Could you check a few things on this drawing? It's one solid part, dimensions in mm from its lowest x, y, z. A direction names the side the tool comes from. Coordinates: 2 decimals unless noted, no trailing zeros. Order: outer loops, then holes, each group sorted by start corner. A loop starts at its lowest first (then second) coordinate and runs counter-clockwise, first axis right, second up. Notation, with made-up numbers: (-6, 48.25) -> (1, 48.25) arc R21 ccw to (1, 58.25) -> close; hole circle Ø4 at (5.5, 3.25). An arc over 180 degrees is marked (long way). Use a Markdown table: item, result. Add a question column.
1. If I drill on line 1 along Z through (x, y) = (36.09, 1.05); line 2 along Y through (x, z) = (40, 22.5), over which ranges is the centre line in solid material (lowest first)? Write a range as from..to.
2. Suppose I cut it at D-D, the plane z = 22.5. List the corners of the cut face in (x, y) for me, then the cut area to 3 significant figures.
3. Suppose I cut it at A-A, the plane z = 6.28. List the corners of the cut face in (x, y) for me, then the cut area to 3 significant figures.
4. Suppose I cut it at C-C, the plane z = 26.5. List the corners of the cut face in (x, y) for me, then the cut area to 3 significant figures.
5. Suppose I cut it at B-B, the plane x = 36.09. List the corners of the cut face in (y, z) for me, then the cut area to 3 significant figures.
6. For pin 1 Ø5 at (x, z) = (19, 13.5) entering from -Y; pin 2 Ø1 at (y, z) = (23, 21) entering from +X; pin 3 Ø1.5 at (x, z) = (27.5, 5) entering from +Y, each with a flat end and sliding along its axis, tell me the tip position at first contact or that it passes through.
7. For the marked faces 1 and 2, which set-ups out of +Z, -Z, +X, -X, +Y, -Y let a thin tool reach every point of the face, with its end or its side?
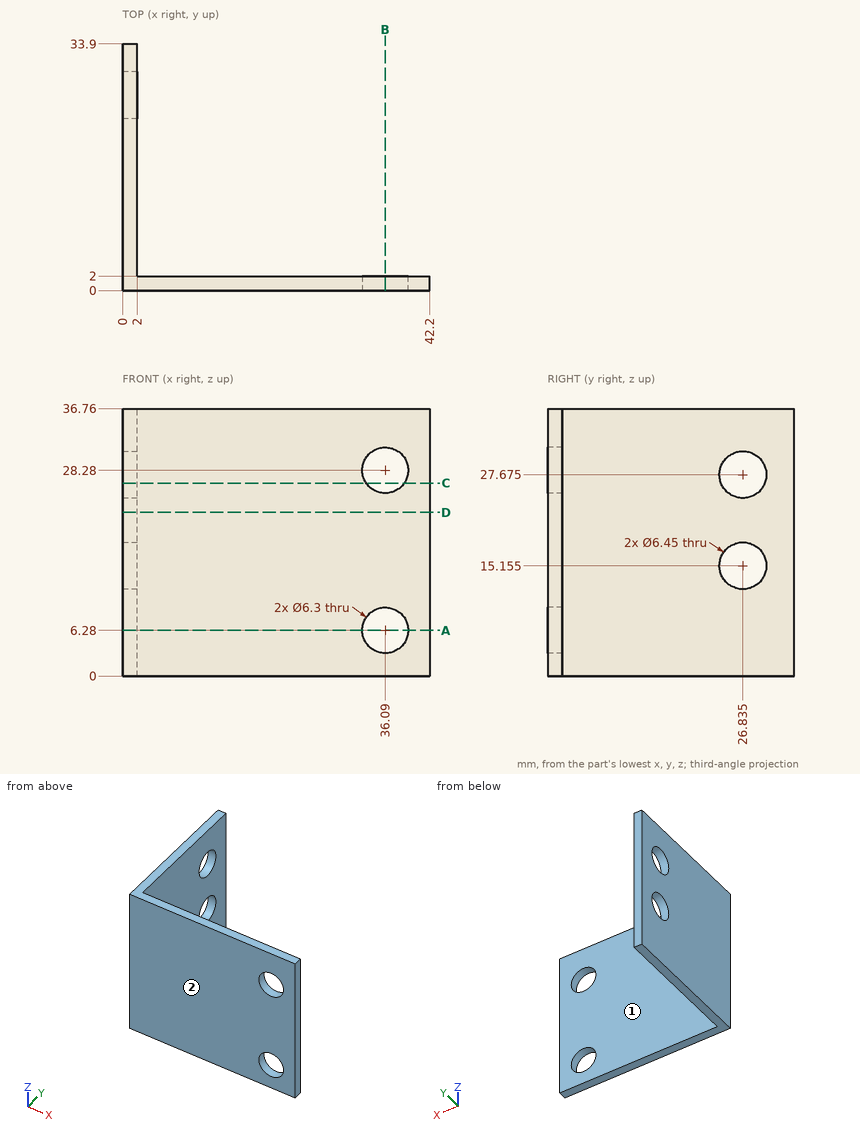
Worked out:
| question | item | result |
|---|---|---|
| 1 | line 1 | z = 0..3.13, 9.43..25.13, 31.43..36.76 |
| 1 | line 2 | y = 0..2 |
| 2 | outline | (0, 0) -> (42.2, 0) -> (42.2, 2) -> (2, 2) -> (2, 33.9) -> (0, 33.9) -> close |
| 2 | area | 148 mm² |
| 3 | outline | (0, 0) -> (32.94, 0) -> (32.94, 2) -> (2, 2) -> (2, 33.9) -> (0, 33.9) -> close; (39.24, 0) -> (42.2, 0) -> (42.2, 2) -> (39.24, 2) -> close |
| 3 | area | 136 mm² |
| 4 | outline | (0, 0) -> (33.49, 0) -> (33.49, 2) -> (2, 2) -> (2, 23.83) -> (0, 23.83) -> close; (0, 29.84) -> (2, 29.84) -> (2, 33.9) -> (0, 33.9) -> close; (38.69, 0) -> (42.2, 0) -> (42.2, 2) -> (38.69, 2) -> close |
| 4 | area | 126 mm² |
| 5 | outline | (0, 0) -> (2, 0) -> (2, 3.13) -> (0, 3.13) -> close; (0, 9.43) -> (2, 9.43) -> (2, 25.13) -> (0, 25.13) -> close; (0, 31.43) -> (2, 31.43) -> (2, 36.76) -> (0, 36.76) -> close |
| 5 | area | 48.3 mm² |
| 6 | pin 1 | stops at y = 0 |
| 6 | pin 2 | stops at x = 2 |
| 6 | pin 3 | stops at y = 2 |
| 7 | face 1 | +Z, -Z, +X, +Y |
| 7 | face 2 | +Z, -Z, +X, -X, -Y |
